CAD build for the part. Positions are in the model's coordinates, mm. A direction names the side the tool comes from. Give positions to 0.01 mm unless a question says otherwise; leave off trailing zeros. Loops run counter-clockwise (first coordinate to the right, second up) from the corner with the lowest first, then second, coordinate; pieces in that order, holes last.
Item 1: Which spindle directions (+Z, -Z, +X, -X, +Y, -Y) get a long thin tool onto all of the face, cutting with end or side? Do faces 4 (the flat face through (-6.744, -58.762, 3.944)), 5 (the cylindrical face through (-9.79, -4.06, 2.46)). Say none if no direction does.
Item 2: Saw through at B-B on y = -36. Give the cut face in (x, z).
Item 3: Mould opens along X. For faces 1 (the cylindrical face through (3.233, -1.341, 6.521)), 2 (the flat face through (18.07, -48.56, 3.94)), 3 (the flat face through (11, -55, 8)) say: released by +X, released by -X, zero draft, split by the parting line, or undercut.
Item 4: Probe probe 1 along Y at (x, z) = (2.5, 6.5); probe 2 along Y at (x, z) = (4, 3.5); probe 3 along Y at (x, z) = (25.5, 4.75). List the from-to ranges inside material, lowest first.
Item 5: Drop flat-ended pins along their axis: P1, Ø17, axis at x = 0, y = 0, coming from the -Z side; P2, Ø2, axis at x = 38, z = 3, coming from the -Y side; P3, Ø1, axis at x = 32, z = 1, coming from the +Y side. Give the stop position or say it passes through.
Item 6: Saw through at A-A on x = 45.5. Give the cut face in (y, z).
from build123d import *

# Parameters (mm, degrees)
SKETCH_1_R          = 14
EXTRUDE_1_DEPTH     = 8
SKETCH_3_R          = 3.5
CUT_EXTRUDE_2_DEPTH = 10
EXTRUDE_START       = -8
EXTRUDE_3_DEPTH     = 8
SKETCH_2_R          = 10.6
CUT_EXTRUDE_3_DEPTH = 5
SKETCH_7_R          = 1.15
CUT_EXTRUDE_4_DEPTH = 5
FILLET_1_R          = 1
FILLET_2_R          = 1


with BuildPart() as part:
    # 스케치1 → 보스-돌출1 (new body)
    with BuildSketch(Plane.XY):
        Circle(SKETCH_1_R)
    extrude(amount=EXTRUDE_1_DEPTH)

    # 스케치3 → 컷-돌출2 (cut)
    with BuildSketch(Plane.XY.offset(8)):
        Circle(SKETCH_3_R)
    extrude(amount=-CUT_EXTRUDE_2_DEPTH, mode=Mode.SUBTRACT)

    # 스케치6 → 보스-돌출3 (add)
    with BuildSketch(Plane.XY.offset(8).offset(EXTRUDE_START)):
        with BuildLine():
            Line((13.735578357, -2.708115061), (22.528484651, -95.708115061))
            ThreePointArc((22.528484651, -95.708115061), (38.172657843, -109.27935171), (52.461884597, -94.288133687))
            ThreePointArc((52.461884597, -94.288133687), (33.515079478, -123.998980013), (0, -113.115264599))
            Line((0, -113.115264599), (-13.64899727, -3.115264599))
            ThreePointArc((-13.64899727, -3.115264599), (0.208126783, -13.998452887), (13.735578357, -2.708115061))
        make_face()
    extrude(amount=EXTRUDE_3_DEPTH)

    # 스케치2 → 컷-돌출3 (cut)
    with BuildSketch(Plane(origin=(0, 0, 0), x_dir=(-1, 0, 0), z_dir=(0, 0, -1))):
        Circle(SKETCH_2_R)
    extrude(amount=-CUT_EXTRUDE_3_DEPTH, mode=Mode.SUBTRACT)

    # 스케치7 → 컷-돌출4 (cut)
    with BuildSketch(Plane(origin=(0, 0, 5), x_dir=(-1, 0, 0), z_dir=(0, 0, -1))):
        with Locations((7, 0)):
            Circle(SKETCH_7_R)
        with Locations((3.5, -6.062177826)):
            Circle(SKETCH_7_R)
        with Locations((-3.5, -6.062177826)):
            Circle(SKETCH_7_R)
        with Locations((-7, 0)):
            Circle(SKETCH_7_R)
        with Locations((-3.5, 6.062177826)):
            Circle(SKETCH_7_R)
        with Locations((3.5, 6.062177826)):
            Circle(SKETCH_7_R)
    extrude(amount=-CUT_EXTRUDE_4_DEPTH, mode=Mode.SUBTRACT)

    # 필렛1
    fillet_1_edges = [part.edges().sort_by_distance(p)[0] for p in [
        (52.461884597, -94.288133687, 4),
    ]]
    fillet(fillet_1_edges, radius=FILLET_1_R)

    # 필렛2
    fillet_2_edges = [part.edges().sort_by_distance(p)[0] for p in [
        (0, -113.115264599, 4),
    ]]
    fillet(fillet_2_edges, radius=FILLET_2_R)


solid = part.part
Results below:
1. face 4: +Z, -Z, -X, -Y
1. face 5: -Z
2. outline: (-9.57, 0) - (16.88, 0) - (16.88, 8) - (-9.57, 8) - close
3. face 1: undercut
3. face 2: released by +X
3. face 3: zero draft
4. probe 1: y = -116.28 to -6.63, -5.49 to -2.45, 2.45 to 5.49, 6.63 to 13.77
4. probe 2: y = -117.81 to -9.82, 9.82 to 13.42
4. probe 3: y = -125.64 to -103.35
5. P1: stops at z = 5
5. P2: stops at y = -122.48
5. P3: stops at y = -108.06
6. outline: (-115.81, 0) - (-106.96, 0) - (-106.96, 8) - (-115.81, 8) - close
